from build123d import *

# Parameters (mm, degrees)
SKETCH_R     = 6.8
PAD_DEPTH    = 0.6
SKETCH001_R  = 4.4
PAD001_DEPTH = 4.8
SKETCH002_R  = 1.75
POCKET_DEPTH = 5
FILLET_R     = 1


with BuildPart() as part:
    # Sketch → Pad (new body)
    with BuildSketch(Plane.XY):
        Circle(SKETCH_R)
    extrude(amount=PAD_DEPTH)

    # Sketch001 (on Face3 of Pad) → Pad001 (join)
    with BuildSketch(Plane.XY.offset(0.6)):
        Circle(SKETCH001_R)
    extrude(amount=PAD001_DEPTH)

    # Sketch002 (on Face2 of Pad001) → Pocket (cut)
    with BuildSketch(Plane(origin=(0, 0, 0), x_dir=(1, 0, 0), z_dir=(0, 0, -1))):
        Circle(SKETCH002_R)
    extrude(amount=-POCKET_DEPTH, mode=Mode.SUBTRACT)

    # Fillet
    fillet_edges = [part.edges().sort_by_distance(p)[0] for p in [
        (-4.4, 0, 5.4),
    ]]
    fillet(fillet_edges, radius=FILLET_R)


solid = part.part
CAD build for the part. Positions are in the model's coordinates, mm. A direction names the side the tool comes from. Round coordinates to 2 decimals unless told otherwise and drop trailing zeros. Order: outer loops, then holes, each group sorted by start corner. A loop starts at its lowest first (then second) coordinate and runs counter-clockwise, first axis right, second up. Notation, with made-up numbers: (40.25, -30) -> (52.25, -30) arc R20 cw to (52.25, -10) -> close; hole circle Ø7 at (7, 48). An arc over 180 degrees is marked (long way). Write item = value, one per line. Start each with the question number.
(1) Which spindle directions (+Z, -Z, +X, -X, +Y, -Y) get a long thin tool onto all of the face, cutting with end or side? Do faces 1 (the flat face through (0, 0, 5.4)), 2 (the flat face through (0, 0, 5)), 3 (the cylindrical face through (4.197, 1.322, 2.473)). Say none if no direction does.
(2) Pin check, flat tips, straight feed: P1, Ø1, axis at y = -2, z = 0.5, coming from the +X side; P2, Ø1, axis at y = 2, z = 3, coming from the -X side. Stop position of each tip, or through.
(3) Pull direction Y, two halves, no side cores. Call faces 4 (the flat face through (1.4, -4.4, 0.6)), 5 (the cylindrical face through (-1.47, -6.64, 0.3)), 6 (the cylindrical face through (1.617, 0.67, 2.465)): released by +Y, released by -Y, zero draft, split by the parting line, or undercut.
(4) Cut at C-C, the plane z = 4. List the corners of the cut face in (x, y).
(5) Probe line 1 (Y direction, x = 0, z = 2); line 2 (Z direction, x = 3.25, y = -4.75); line 3 (Y direction, x = -1.5, z = 4.25). List the from-to ranges inside material, lowest first. Write a range as [from, to].
(6) Cut at A-A, the plane y = 0. List the corners of the cut face in (x, z).
(7) Cut at D-D, the plane y = -6. List the corners of the cut face in (x, z), then the cut area to 3 significant figures.
Model answer:
q1.face_1 = +Z, +X, -X, +Y, -Y
q1.face_2 = -Z
q1.face_3 = +Z
q2.P1 = 6.63
q2.P2 = -4.14
q3.face_4 = zero draft
q3.face_5 = split by the parting line
q3.face_6 = undercut
q4.outline = circle Ø8.8 at (0, 0); hole circle Ø3.5 at (0, 0)
q5.line_1 = [-4.4, -1.75], [1.75, 4.4]
q5.line_2 = [0, 0.6]
q5.line_3 = [-4.14, -0.9], [0.9, 4.14]
q6.outline = (-6.8, 0) -> (-1.75, 0) -> (-1.75, 5) -> (1.75, 5) -> (1.75, 0) -> (6.8, 0) -> (6.8, 0.6) -> (4.4, 0.6) -> (4.4, 4.4) arc R1 ccw to (3.4, 5.4) -> (-3.4, 5.4) arc R1 ccw to (-4.4, 4.4) -> (-4.4, 0.6) -> (-6.8, 0.6) -> close
q7.outline = (-3.2, 0) -> (3.2, 0) -> (3.2, 0.6) -> (-3.2, 0.6) -> close
q7.area = 3.84 mm2
